Geometry: see drawing. Coordinates: mm, zero at the bounding-box minimum. A direction names the side the tool comes from. Round coordinates to 2 decimals unless told otherwise and drop trailing zeros. Order: outer loops, then holes, each group sorted by start corner. A loop starts at its lowest first (then second) coordinate and runs counter-clockwise, first axis right, second up. Notation, with made-up numbers: (76, 65) -> (116, 65) arc R20 cw to (116, 87) -> close; hole circle Ø5 at (-34, 69.5). An arc over 180 degrees is marked (long way). Use a Markdown table: item, result.
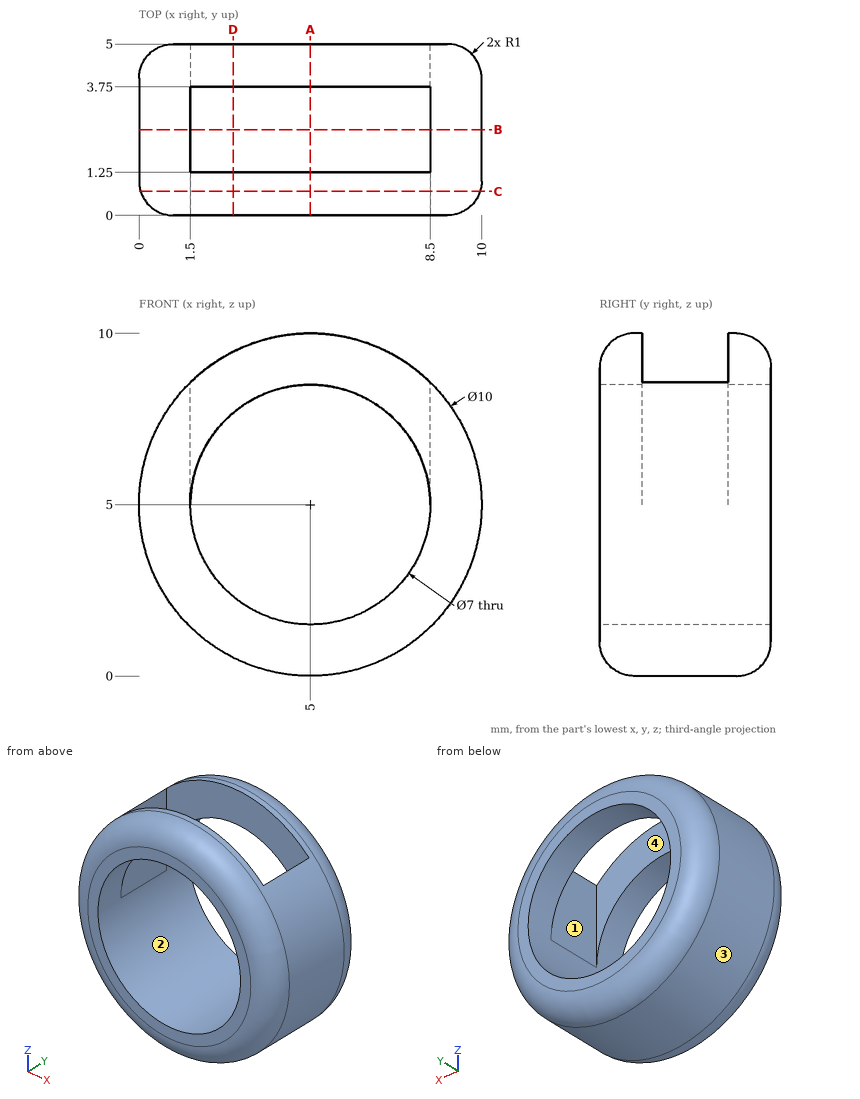
1) Cut plane C-C on y = 0.7. Return loops of the section in (x, z).
Answer key:
| item | result |
|---|---|
| outline | circle Ø9.91 at (5, 5); hole circle Ø7 at (5, 5) |
2) Cut plane A-A on x = 5. Return loops of the section in (y, z).
Answer key:
| item | result |
|---|---|
| outline | (0, 1) arc R1 ccw to (1, 0) -> (4, 0) arc R1 ccw to (5, 1) -> (5, 1.5) -> (0, 1.5) -> close; (0, 8.5) -> (1.25, 8.5) -> (1.25, 10) -> (1, 10) arc R1 ccw to (0, 9) -> close; (3.75, 8.5) -> (5, 8.5) -> (5, 9) arc R1 ccw to (4, 10) -> (3.75, 10) -> close |
3) Cut plane D-D on x = 2.75. State how many separate pieces and enclosed holes the cut face has, and give its area (3 significant figures).
Answer key:
| item | result |
|---|---|
| separate pieces | 3 |
| enclosed holes | 0 |
| area | 12.4 mm^2 |
4) Contact query for flat-ended pins moving along their axis: P1, Ø4, axis at x = 4.5, z = 6.5, coming from the -Y side; P2, Ø1.2, axis at y = 2.5, z = 7.5, coming from the -X side. Output: stop coordinate, or through.
Answer key:
| item | result |
|---|---|
| P1 | stops at y = 0 |
| P2 | stops at x = 0.38 |
5) Ray query, probe 1 along Z at (x, y) = (5, 1.05); probe 2 along Z at (x, y) = (5, 2.35). Return the intervals inside material, ascending.
Answer key:
| item | result |
|---|---|
| probe 1 | z = 0 to 1.5, 8.5 to 10 |
| probe 2 | z = 0 to 1.5 |
6) Draft query along Y for the marked faces 1 and 2. Return one class per face: released by +Y, released by -Y, zero draft, split by the parting line, or undercut.
Answer key:
| item | result |
|---|---|
| face 1 | undercut |
| face 2 | zero draft |
7) Cut plane B-B on y = 2.5. Return loops of the section in (x, z), and give its area (3 significant figures).
Answer key:
| item | result |
|---|---|
| outline | (1.5, 5) -> (1.5, 8.57) arc R5 ccw (long way) to (8.5, 8.57) -> (8.5, 5) arc R3.5 cw to start |
| area | 27.4 mm^2 |
8) Set-up query: the marked faces 3 and 4. Return all of +Z, -Z, +X, -X, +Y, -Y with unobstructed straight access to the full face (end or side cutting, diameter ignored); none if empty.
Answer key:
| item | result |
|---|---|
| face 3 | +Y, -Y |
| face 4 | +Z |
